The model under review builds one solid part; all positions refer to its coordinate system, in mm. A direction names the side the tool comes from. Give positions to 0.01 mm unless a question says otherwise; leave off trailing zeros. Loops run counter-clockwise (first coordinate to the right, second up) from the corner with the lowest first, then second, coordinate; pieces in that order, holes last. Notation, with made-up numbers: (35, 60.5) -> (79, 60.5) arc R26 ccw to (79, 77.5) -> close; hole circle Ø4 at (-18, 53). An arc over 180 degrees is marked (long way). Write each question's results on one line, items separated by ' | '. Start each with the question number.
Q1. We need section A-A (y = -9.5). Write out the cut boundary in (x, z).
Q2. Wall thickness on L1, parallel to Z at x = -21.25, y = 28.95; L2, parallel to Y at x = -35.75, z = 9.25; L3, parallel to Y at x = 33.5, z = 11.75: over which ranges is each line inside the solid? List them lowest first. Write a range as [from, to].
Q3. Insertion check: pin 1 Ø1.5 at (x, y) = (-34.5, -11.5) entering from -Z; pin 2 Ø1.6 at (x, y) = (40.75, 26.5) entering from -Z; pin 3 Ø2.5 at (x, y) = (-35.75, 26.5) entering from -Z. Each pin has a flat end and moves straight along its axis. Give the tip position at first contact, or say it passes through.
Q4. We need section D-D (y = -2). Write out the cut boundary in (x, z), plus the area to 3 significant figures.
Q5. Machinability: for faces 1 (the face through (-36.25, 0, 4)), 2 (the face through (-28, 28, 6)), 3 (the face through (-36.29, -27.66, 7.15)), which of the approach directions +Z, -Z, +X, -X, +Y, -Y give a long, thin tool a straight path to every point of the face, cutting with its end or side? Answer none if there is none.
Q6. We need section B-B (x = -26). Write out the cut boundary in (y, z).
Q7. We need section C-C (z = 8). Give the number of separate pieces and of enclosed holes in the cut face, plus the area to 3 significant figures.
Q8. Mouldability with a two-part tool opening along X and no side actions: class faces 4 (the face through (14, -28, 0)), 5 (the face through (31, 24, 10)), 6 (the face through (-38.25, -1, 8)) as released by +X, released by -X, zero draft, split by the parting line, or undercut.
from build123d import *

# Parameters (mm, degrees)
SKETCH1_W             = 81.5
SKETCH1_H             = 60
BOSS_EXTRUDE1_DEPTH   = 14
SKETCH3_W             = 81.5
SKETCH3_H             = 60
BOSS_EXTRUDE2_DEPTH   = 2
SKETCH4_R             = 3.25
CUT_EXTRUDE1_DEPTH    = 2
SKETCH5_R             = 1.875
CUT_EXTRUDE2_DEPTH    = 2
SKETCH6_R             = 0.9
BOSS_EXTRUDE3_DEPTH   = 9
BOSS_EXTRUDE4_DEPTH   = 9
FILLET1_R             = 3
SKETCH9_R             = 1
CUT_EXTRUDE3_DEPTH    = 17
CHAMFER1_SIZE         = 1.5
CHAMFER1_SIZE2        = 1.050311307
CHAMFER1_PART_2_SIZE  = 1.5
CHAMFER1_PART_2_SIZE2 = 1.050311307
CHAMFER1_PART_3_SIZE  = 1.5
CHAMFER1_PART_3_SIZE2 = 1.050311307
CHAMFER1_PART_4_SIZE  = 1.5
CHAMFER1_PART_4_SIZE2 = 1.050311307
CUT_EXTRUDE4_REACH    = 62
SKETCH10_W            = 6
SKETCH10_H            = 6
CHAMFER2_SIZE         = 1
SKETCH11_R            = 2.5
SKETCH11_R_2          = 1.25
SKETCH11_W            = 1.5
SKETCH11_H            = 5
CUT_EXTRUDE5_DEPTH    = 0.5


with BuildPart() as part:
    # Sketch1 → Boss-Extrude1 (new body)
    with BuildSketch(Plane.XY):
        with Locations((2.5, -1)):
            Rectangle(SKETCH1_W, SKETCH1_H)
        with BuildLine():
            Line((-36.25, -27), (-36.25, 24.25))
            ThreePointArc((-36.25, 24.25), (-34.218257349, 24.968257349), (-33.5, 27))
            Line((-33.5, 27), (38.5, 27))
            ThreePointArc((38.5, 27), (39.218257349, 24.968257349), (41.25, 24.25))
            Line((41.25, 24.25), (41.25, -27))
            Line((41.25, -27), (-36.25, -27))
        make_face(mode=Mode.SUBTRACT)
    extrude(amount=BOSS_EXTRUDE1_DEPTH)

    # Sketch3 → Boss-Extrude2 (add)
    with BuildSketch(Plane.XY.offset(14)):
        with Locations((2.5, -1)):
            Rectangle(SKETCH3_W, SKETCH3_H)
    extrude(amount=BOSS_EXTRUDE2_DEPTH)

    # Sketch4 → Cut-Extrude1 (cut)
    with BuildSketch(Plane.ZY.offset(38.25)):
        with Locations((0.5, -18)):
            Circle(SKETCH4_R)
        with Locations((0.5, -2)):
            Circle(SKETCH4_R)
        with Locations((0.5, 14)):
            Circle(SKETCH4_R)
    extrude(amount=-CUT_EXTRUDE1_DEPTH, mode=Mode.SUBTRACT)

    # Sketch5 → Cut-Extrude2 (cut)
    with BuildSketch(Plane(origin=(0, 29, 0), x_dir=(1, 0, 0), z_dir=(0, 1, 0))):
        with Locations((8, 0.5)):
            Circle(SKETCH5_R)
        with Locations((-1.7, 0.5)):
            Circle(SKETCH5_R)
    extrude(amount=-CUT_EXTRUDE2_DEPTH, mode=Mode.SUBTRACT)

    # Sketch6 → Boss-Extrude3 (add)
    with BuildSketch(Plane(origin=(0, 0, 14), x_dir=(-1, 0, 0), z_dir=(0, 0, -1))):
        with BuildLine():
            Line((-31, -24.25), (-31, -27))
            Line((-31, -27), (-41.25, -27))
            Line((-41.25, -27), (-41.25, -21.75))
            Line((-41.25, -21.75), (-33.5, -21.75))
            ThreePointArc((-33.5, -21.75), (-31.732233047, -22.482233047), (-31, -24.25))
        make_face()
        with Locations((-33.5, -24.25)):
            Circle(SKETCH6_R, mode=Mode.SUBTRACT)
        with BuildLine():
            Line((-41.25, 19.25), (-33.5, 19.25))
            ThreePointArc((-33.5, 19.25), (-31.732233047, 19.982233047), (-31, 21.75))
            Line((-31, 21.75), (-31, 27))
            Line((-31, 27), (-41.25, 27))
            Line((-41.25, 27), (-41.25, 19.25))
        make_face()
        with Locations((-33.5, 21.75)):
            Circle(SKETCH6_R, mode=Mode.SUBTRACT)
    extrude(amount=BOSS_EXTRUDE3_DEPTH)

    # Sketch7 → Boss-Extrude4 (add)
    with BuildSketch(Plane(origin=(0, 0, 14), x_dir=(-1, 0, 0), z_dir=(0, 0, -1))):
        Polygon((36.25, -27), (34.25, -27), (34.25, 24), (33.25, 24), (33.25, 27), (36.25, 27), align=None)
    extrude(amount=BOSS_EXTRUDE4_DEPTH)

    # Fillet1
    fillet1_edges = [part.edges().sort_by_distance(p)[0] for p in [
        (41.25, -27, 2.5),
        (-36.25, -27, 2.5),
    ]]
    fillet(fillet1_edges, radius=FILLET1_R)

    # Sketch9 → Cut-Extrude3 (cut, through all)
    with BuildSketch(Plane(origin=(0, 0, 0), x_dir=(-1, 0, 0), z_dir=(0, 0, -1))):
        with Locations((35.75, -28.5)):
            Circle(SKETCH9_R)
        with Locations((-40.75, -28.5)):
            Circle(SKETCH9_R)
        with Locations((-40.75, 26.5)):
            Circle(SKETCH9_R)
        with Locations((35.75, 26.5)):
            Circle(SKETCH9_R)
    extrude(amount=-CUT_EXTRUDE3_DEPTH, mode=Mode.SUBTRACT)

    # Chamfer1
    chamfer1_edges = [part.edges().sort_by_distance(p)[0] for p in [
        (-34.75, 26.5, 16),
    ]]
    chamfer1_side = [part.faces().sort_by_distance(p)[0] for p in [
        (-34.75, 26.5, 8),
    ]]
    chamfer(chamfer1_edges, length=CHAMFER1_SIZE, length2=CHAMFER1_SIZE2, reference=chamfer1_side[0])

    # Chamfer1 part 2
    chamfer1_part_2_edges = [part.edges().sort_by_distance(p)[0] for p in [
        (41.75, 26.5, 16),
    ]]
    chamfer1_part_2_side = [part.faces().sort_by_distance(p)[0] for p in [
        (41.75, 26.5, 8),
    ]]
    chamfer(chamfer1_part_2_edges, length=CHAMFER1_PART_2_SIZE, length2=CHAMFER1_PART_2_SIZE2, reference=chamfer1_part_2_side[0])

    # Chamfer1 part 3
    chamfer1_part_3_edges = [part.edges().sort_by_distance(p)[0] for p in [
        (41.75, -28.5, 16),
    ]]
    chamfer1_part_3_side = [part.faces().sort_by_distance(p)[0] for p in [
        (41.75, -28.5, 8),
    ]]
    chamfer(chamfer1_part_3_edges, length=CHAMFER1_PART_3_SIZE, length2=CHAMFER1_PART_3_SIZE2, reference=chamfer1_part_3_side[0])

    # Chamfer1 part 4
    chamfer1_part_4_edges = [part.edges().sort_by_distance(p)[0] for p in [
        (-34.75, -28.5, 16),
    ]]
    chamfer1_part_4_side = [part.faces().sort_by_distance(p)[0] for p in [
        (-34.75, -28.5, 8),
    ]]
    chamfer(chamfer1_part_4_edges, length=CHAMFER1_PART_4_SIZE, length2=CHAMFER1_PART_4_SIZE2, reference=chamfer1_part_4_side[0])

    # Sketch10 → Cut-Extrude4 (cut, up to next)
    with BuildSketch(Plane(origin=(0, 29, 0), x_dir=(1, 0, 0), z_dir=(0, 1, 0)), mode=Mode.PRIVATE) as cut_extrude4_sk1:
        with Locations((-27.9, -3)):
            Rectangle(SKETCH10_W, SKETCH10_H)
    cut_extrude4_tool1 = extrude(cut_extrude4_sk1.sketch, amount=-CUT_EXTRUDE4_REACH, mode=Mode.PRIVATE) & part.part
    add(cut_extrude4_tool1.solids().sort_by_distance((-27.9, 29, 3))[0], mode=Mode.SUBTRACT)

    # Chamfer2
    chamfer2_edges = [part.edges().sort_by_distance(p)[0] for p in [
        (-38.25, -18, 3.75),
        (-38.25, -2, 3.75),
        (-38.25, 14, 3.75),
    ]]
    chamfer(chamfer2_edges, length=CHAMFER2_SIZE)

    # Sketch11 → Cut-Extrude5 (cut)
    with BuildSketch(Plane(origin=(0, 29, 0), x_dir=(1, 0, 0), z_dir=(0, 1, 0))):
        with Locations((-21.25, -8)):
            Circle(SKETCH11_R)
        with Locations((-21.25, -8)):
            Circle(SKETCH11_R_2, mode=Mode.SUBTRACT)
        with Locations((-33.5, -8)):
            Rectangle(SKETCH11_W, SKETCH11_H)
    extrude(amount=-CUT_EXTRUDE5_DEPTH, mode=Mode.SUBTRACT)


solid = part.part
Output:
1) outline: (-38.25, 0) -> (-36.25, 0) -> (-36.25, 5) -> (-34.25, 5) -> (-34.25, 14) -> (41.25, 14) -> (41.25, 0) -> (43.25, 0) -> (43.25, 16) -> (-38.25, 16) -> close
2) L1: [0, 5.5], [6.75, 9.25], [10.5, 16] | L2: [-31, -29.5], [-27.5, 25.5], [27.5, 29] | L3: [-31, -25.15], [-23.35, -21.75], [19.25, 20.85], [22.65, 29]
3) pin 1: z = 5 | pin 2: through | pin 3: z = 0
4) outline: (-38.25, 4.75) -> (-37.25, 3.75) -> (-36.25, 3.75) -> (-36.25, 5) -> (-34.25, 5) -> (-34.25, 14) -> (41.25, 14) -> (41.25, 0) -> (43.25, 0) -> (43.25, 16) -> (-38.25, 16) -> close | area: 229 mm2
5) face 1: -Z | face 2: -Z, +Y | face 3: +Z, -Z
6) outline: (-31, 0) -> (-27, 0) -> (-27, 14) -> (27, 14) -> (27, 6) -> (29, 6) -> (29, 16) -> (-31, 16) -> close
7) separate pieces: 1 | enclosed holes: 7 | area: 927 mm2
8) face 4: zero draft | face 5: undercut | face 6: released by -X
